The model under review builds one solid part; all positions refer to its coordinate system, in mm. A direction names the side the tool comes from. Coordinates: 2 decimals unless noted, no trailing zeros. Order: outer loops, then holes, each group sorted by start corner. A loop starts at its lowest first (then second) coordinate and runs counter-clockwise, first axis right, second up.
```python
from build123d import *

# Parameters (mm, degrees)
SKETCH_1_W                        = 240
SKETCH_1_H                        = 125
EXTRUDE_1_DEPTH                   = 4
HOLE_WIZARD_5_4_5_4_1_D           = 5.4
HOLE_WIZARD_5_4_5_4_1_CSINK_D     = 5.45
HOLE_WIZARD_5_4_5_4_1_CSINK_ANGLE = 90
FILLET_1_R                        = 3
SKETCH_5_R                        = 10
EXTRUDE_2_DEPTH                   = 6
EXTRUDE_START                     = 14.5
EXTRUDE_3_DEPTH                   = 3
FILLET_2_R                        = 3
SKETCH_8_W                        = 6.5
SKETCH_8_H                        = 20
EXTRUDE_4_DEPTH                   = 8
SKETCH_10_R                       = 2
CUT_EXTRUDE_1_DEPTH               = 148.296469747
SKETCH_11_R                       = 5.486659136
EXTRUDE_5_DEPTH                   = 7


with BuildPart() as part:
    # 草图1 → 凸台-拉伸1 (new body)
    with BuildSketch(Plane(origin=(0, 0, 0), x_dir=(1, 0, 0), z_dir=(0, 1, 0))):
        Rectangle(SKETCH_1_W, SKETCH_1_H)
    extrude(amount=EXTRUDE_1_DEPTH)

    # Ø5.4 (5.4) 直径孔1 (through all)
    with Locations(Plane(origin=(0, 4, 0), x_dir=(1, 0, 0), z_dir=(0, 1, 0))):
        with Locations((112, 54.5), (-112, 54.5), (-112, -54.5), (112, -54.5)):
            CounterSinkHole(HOLE_WIZARD_5_4_5_4_1_D / 2, HOLE_WIZARD_5_4_5_4_1_CSINK_D / 2, counter_sink_angle=HOLE_WIZARD_5_4_5_4_1_CSINK_ANGLE)

    # 圆角1
    fillet_1_edges = [part.edges().sort_by_distance(p)[0] for p in [
        (120, 2, 62.5),
        (-120, 2, 62.5),
        (-120, 2, -62.5),
        (120, 2, -62.5),
    ]]
    fillet(fillet_1_edges, radius=FILLET_1_R)

    # 草图5 → 凸台-拉伸2 (add)
    with BuildSketch(Plane.XY):
        with BuildLine():
            Line((-60, 4), (-39.5, 4))
            Line((-39.5, 4), (-39.5, 16))
            Line((-39.5, 16), (-33, 16))
            Line((-33, 16), (-33, 36))
            Line((-33, 36), (-43.116750419, 36))
            ThreePointArc((-43.116750419, 36), (-49.75, 38), (-56.383249581, 36))
            Line((-56.383249581, 36), (-87, 36))
            Line((-87, 36), (-87, 16))
            Line((-87, 16), (-60, 16))
            Line((-60, 16), (-60, 4))
        make_face()
        with Locations((-49.75, 26)):
            Circle(SKETCH_5_R, mode=Mode.SUBTRACT)
    extrude(amount=EXTRUDE_2_DEPTH)

    # 草图6 → 凸台-拉伸3 (add)
    with BuildSketch(Plane(origin=(0, 0, 0), x_dir=(-1, 0, 0), z_dir=(0, 0, -1)).offset(EXTRUDE_START)):
        with BuildLine():
            Line((39.5, 4), (60, 4))
            Line((60, 4), (60, 32.239991987))
            ThreePointArc((60, 32.239991987), (49.75, 38), (39.5, 32.239991987))
            Line((39.5, 32.239991987), (39.5, 4))
        make_face()
    extrude(amount=-EXTRUDE_3_DEPTH)

    # 圆角2
    fillet_2_edges = [part.edges().sort_by_distance(p)[0] for p in [
        (-49.75, 4, -11.5),
        (-49.75, 4, -14.5),
    ]]
    fillet(fillet_2_edges, radius=FILLET_2_R)

    # 草图8 → 凸台-拉伸4 (add)
    with BuildSketch(Plane.XY.offset(6)):
        with Locations((-36.25, 26)):
            Rectangle(SKETCH_8_W, SKETCH_8_H)
        with Locations((-83.75, 26)):
            Rectangle(SKETCH_8_W, SKETCH_8_H)
    extrude(amount=EXTRUDE_4_DEPTH)

    # 草图10 → 切除-拉伸1 (cut, through all)
    with BuildSketch(Plane.XY.offset(14)):
        with Locations((-83.75, 31)):
            Circle(SKETCH_10_R)
        with Locations((-83.75, 21)):
            Circle(SKETCH_10_R)
        with Locations((-36.25, 21)):
            Circle(SKETCH_10_R)
        with Locations((-36.25, 31)):
            Circle(SKETCH_10_R)
    extrude(amount=-CUT_EXTRUDE_1_DEPTH, mode=Mode.SUBTRACT)

    # 草图11 → 凸台-拉伸5 (add)
    with BuildSketch(Plane(origin=(0, 0, -14.5), x_dir=(-1, 0, 0), z_dir=(0, 0, -1))):
        with Locations((49.501785155, 27.302934709)):
            Circle(SKETCH_11_R)
    extrude(amount=-EXTRUDE_5_DEPTH)


solid = part.part
```
(1) We need section C-C, the plane x = 58.5. Write out the cut boundary in (y, z).
A:
outline: (0, -62.5) - (4, -62.5) - (4, 62.5) - (0, 62.5) - close
(2) We need section B-B, the plane z = -54.5. Write out the cut boundary in (x, y) (3 decimals).
A:
outline: (-120, 0) - (-114.7, 0) - (-114.7, 3.975) - (-114.725, 4) - (-120, 4) - close; (-109.3, 0) - (109.3, 0) - (109.3, 3.975) - (109.275, 4) - (-109.275, 4) - (-109.3, 3.975) - close; (114.7, 0) - (120, 0) - (120, 4) - (114.725, 4) - (114.7, 3.975) - close
(3) Draft analysis for pull direction X (two halves, no side actions). For faces 4 (the face through (-36, 26, 14)), 5 (the face through (-49.9, 38, -13)), 6 (the face through (-60, 21, 6)), state which applies: released by +X, released by -X, zero draft, split by the parting line, or undercut.
A:
face 4: zero draft
face 5: split by the parting line
face 6: undercut
(4) For pin 1 Ø3.5 at (x, y) = (-83.75, 21) entering from +Z; pin 2 Ø9 at (y, z) = (27.5, 11) entering from -X; pin 3 Ø4 at (x, z) = (11, 10) entering from +Y; pin 4 Ø3.5 at (x, y) = (-47.5, 25) entering from +Z, all flat-tipped, find the tip position at first contact; note any pin that passes through.
A:
pin 1: passes through
pin 2: stops at x = -87
pin 3: stops at y = 4
pin 4: stops at z = -7.5
(5) Wall thickness on probe 1 along X at (y, z) = (2.55, 54.5); probe 2 along Y at (x, z) = (-83.75, 5.25); probe 3 along Y at (x, z) = (-85.5, 1): over which ranges is each line inside the solid? List them lowest first.
A:
probe 1: x = -120 to -114.7, -109.3 to 109.3, 114.7 to 120
probe 2: y = 0 to 4, 16 to 19, 23 to 29, 33 to 36
probe 3: y = 0 to 4, 16 to 20.03, 21.97 to 30.03, 31.97 to 36
(6) Machinability: for faces 1 (the face through (-77, 16, 4)), 2 (the face through (-37, 36, 7)), 3 (the face through (-45.15, 23.96, -9.53)), which of the approach directions +Z, -Z, +X, -X, +Y, -Y give a long, thin tool a straight path to every point of the face, cutting with its end or side? Answer none if there is none.
A:
face 1: +Z, -Z, -X
face 2: +Z, -Z, +X, +Y
face 3: +Z
(7) We need section D-D, the plane z = 30. Write out the cut boundary in (x, y), and give its area (3 significant figures).
A:
outline: (-120, 0) - (120, 0) - (120, 4) - (-120, 4) - close
area: 960 mm2
(8) We need section A-A, the plane x = 112. Write out the cut boundary in (y, z) (3 decimals), and give its area (3 significant figures).
A:
outline: (0, -62.5) - (4, -62.5) - (4, -57.225) - (3.975, -57.2) - (0, -57.2) - close; (0, -51.8) - (3.975, -51.8) - (4, -51.775) - (4, 51.775) - (3.975, 51.8) - (0, 51.8) - close; (0, 57.2) - (3.975, 57.2) - (4, 57.225) - (4, 62.5) - (0, 62.5) - close
area: 457 mm2
